Build history of the part. All positions in model axes, mm. Face numbers are marked on the shaded views. A direction names the side the tool comes from. Give positions to 0.01 mm unless a question says otherwise; leave off trailing zeros. Loops run counter-clockwise (first coordinate to the right, second up) from the corner with the lowest first, then second, coordinate; pieces in that order, holes last. Notation, with made-up numbers: (-39, 27) -> (-20, 27) arc R19 ccw to (-20, 63) -> close; hole circle Ø1 at (38, 52.5). An arc over 180 degrees is marked (long way). Answer in a Markdown table with one row per item. Add a question column.
from build123d import *

# Parameters (mm, degrees)
SKETCH1_W           = 43.20032
SKETCH1_H           = 28.39974
BOSS_EXTRUDE1_DEPTH = 13.4747
SKETCH2_W           = 33.20034
SKETCH2_H           = 20.39874
CUT_EXTRUDE1_DEPTH  = 10.2997
SKETCH3_W           = 5.19938
SKETCH3_H           = 12.10056
CUT_EXTRUDE2_DEPTH  = 53.715241631


with BuildPart() as part:
    # Sketch1 → Boss-Extrude1 (new body)
    with BuildSketch(Plane(origin=(0, 0, 0), x_dir=(1, 0, 0), z_dir=(0, 1, 0))):
        with Locations((21.60016, 14.19987)):
            Rectangle(SKETCH1_W, SKETCH1_H)
    extrude(amount=BOSS_EXTRUDE1_DEPTH)

    # Sketch2 → Cut-Extrude1 (cut)
    with BuildSketch(Plane(origin=(0, 13.4747, 0), x_dir=(1, 0, 0), z_dir=(0, 1, 0))):
        with Locations((26.60015, 14.19987)):
            Rectangle(SKETCH2_W, SKETCH2_H)
    extrude(amount=-CUT_EXTRUDE1_DEPTH, mode=Mode.SUBTRACT)

    # Sketch3 → Cut-Extrude2 (cut, through all)
    with BuildSketch(Plane(origin=(0, 3.175, 0), x_dir=(1, 0, 0), z_dir=(0, 1, 0))):
        with Locations((17.60093, 14.19987)):
            Rectangle(SKETCH3_W, SKETCH3_H)
    extrude(amount=-CUT_EXTRUDE2_DEPTH, mode=Mode.SUBTRACT)


solid = part.part
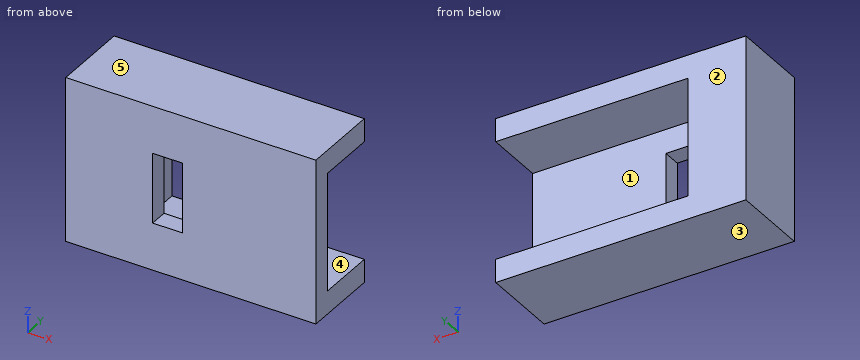
(1) Wall check: line 1 along Z through (x, y) = (29.5, 7.5); line 2 along Z through (x, y) = (20, 1.75); line 3 along Y through (x, z) = (36.5, -18) (3 decimals). Give the ranges that are in metal, low to high. Write a range as from..to.
(2) Saw through at A-A, the plane x = 15.5. List the corners of the cut face in (y, z) (1 decimal).
(3) Two-plate mould, pull along Z, no slides. Class the marked faces 3, 4 and 5: released by +Z, released by -Z, zero draft, split by the parting line, or undercut.
(4) Flat gauge pins, fed straight in: pin 1 Ø6 at (x, z) = (33, -12) entering from +Y (3 decimals); pin 2 Ø5 at (y, z) = (9.5, -14.5) entering from +X. Where does each tip first touch, or does it go through?
(5) 3-axis set-ups, long thin cutter, end or side, ignore diameter. For the marked faces 1 and 2: which of +Z, -Z, +X, -X, +Y, -Y reach the whole face in a straight line?
(6) Saw through at C-C, the plane x = 30. List the corners of the cut face in (y, z) (1 decimal).
(7) Saw through at B-B, the plane z = -9. List the corners of the cut face in (x, y) (3 decimals).
(8) Saw through at D-D, the plane y = 1.5. List the corners of the cut face in (x, z), then the cut area to 3 significant figures.
Worked answers:
| question | item | result |
|---|---|---|
| 1 | line 1 | -28.4..-24.4, -4..0 |
| 1 | line 2 | -28.4..-20.25, -8.15..0 |
| 1 | line 3 | 0..3.175 |
| 2 | outline | (0, -28.4) -> (13.5, -28.4) -> (13.5, -24.4) -> (3.2, -24.4) -> (3.2, -20.3) -> (0, -20.3) -> close; (0, -8.1) -> (3.2, -8.1) -> (3.2, -4) -> (13.5, -4) -> (13.5, 0) -> (0, 0) -> close |
| 3 | face 3 | released by -Z |
| 3 | face 4 | undercut |
| 3 | face 5 | released by +Z |
| 4 | pin 1 | y = 3.175 |
| 4 | pin 2 | x = 10 |
| 5 | face 1 | +X, +Y |
| 5 | face 2 | +Z, -Z, +X, -X, +Y |
| 6 | outline | (0, -28.4) -> (13.5, -28.4) -> (13.5, -24.4) -> (3.2, -24.4) -> (3.2, -4) -> (13.5, -4) -> (13.5, 0) -> (0, 0) -> close |
| 7 | outline | (0, 0) -> (15.001, 0) -> (15.001, 3.175) -> (10, 3.175) -> (10, 13.475) -> (0, 13.475) -> close; (20.201, 0) -> (43.2, 0) -> (43.2, 3.175) -> (20.201, 3.175) -> close |
| 8 | outline | (0, -28.4) -> (43.2, -28.4) -> (43.2, 0) -> (0, 0) -> close; hole (15, -20.25) -> (20.2, -20.25) -> (20.2, -8.15) -> (15, -8.15) -> close |
| 8 | area | 1,160 mm^2 |
